```python
from build123d import *

# Parameters (mm, degrees)
SKETCH1_W           = 393.4
SKETCH1_H           = 150
BOSS_EXTRUDE1_DEPTH = 3.3
SKETCH2_R           = 2
CUT_EXTRUDE1_DEPTH  = 257.520622953
SKETCH3_R           = 2
CUT_EXTRUDE2_DEPTH  = 4
SKETCH4_R           = 2
CUT_EXTRUDE3_DEPTH  = 4
SKETCH6_W           = 29.5
SKETCH6_H           = 13
SKETCH6_W_2         = 121.579447476
SKETCH6_H_2         = 18.9
CUT_EXTRUDE4_DEPTH  = 10


with BuildPart() as part:
    # Sketch1 → Boss-Extrude1 (new body)
    with BuildSketch(Plane.XY):
        with Locations((27, -50.5)):
            Rectangle(SKETCH1_W, SKETCH1_H)
    extrude(amount=BOSS_EXTRUDE1_DEPTH)

    # Sketch2 → Cut-Extrude1 (cut, through all)
    with BuildSketch(Plane(origin=(0, 0, 0), x_dir=(-1, 0, 0), z_dir=(0, 0, -1))):
        with Locations((-183.7, -115.5)):
            Circle(SKETCH2_R)
        with Locations((-213.7, -115.5)):
            Circle(SKETCH2_R)
        with Locations((129.7, -115.5)):
            Circle(SKETCH2_R)
        with Locations((159.7, -115.5)):
            Circle(SKETCH2_R)
    extrude(amount=-CUT_EXTRUDE1_DEPTH, mode=Mode.SUBTRACT)

    # Sketch3 → Cut-Extrude2 (cut)
    with BuildSketch(Plane.XY.offset(3.3)):
        with Locations((-159.7, 14.5)):
            Circle(SKETCH3_R)
        with Locations((-139.7, 14.5)):
            Circle(SKETCH3_R)
        with Locations((193.7, 14.5)):
            Circle(SKETCH3_R)
        with Locations((213.7, 14.5)):
            Circle(SKETCH3_R)
    extrude(amount=-CUT_EXTRUDE2_DEPTH, mode=Mode.SUBTRACT)

    # Sketch4 → Cut-Extrude3 (cut)
    with BuildSketch(Plane.XY.offset(3.3)):
        with Locations((12, 12.25)):
            Circle(SKETCH4_R)
        with Locations((42, 12.25)):
            Circle(SKETCH4_R)
    extrude(amount=-CUT_EXTRUDE3_DEPTH, mode=Mode.SUBTRACT)

    # Sketch6 → Cut-Extrude4 (cut)
    with BuildSketch(Plane(origin=(0, 0, 0), x_dir=(-1, 0, 0), z_dir=(0, 0, -1))):
        with Locations((-36.8, -79)):
            Rectangle(SKETCH6_W, SKETCH6_H)
        with Locations((-27, -97.742382112)):
            Rectangle(SKETCH6_W_2, SKETCH6_H_2)
    extrude(amount=-CUT_EXTRUDE4_DEPTH, mode=Mode.SUBTRACT)


solid = part.part
```
Geometry: final body of the model. Coordinates: model frame, mm. Round coordinates to 2 decimals unless told otherwise and drop trailing zeros. Loops run counter-clockwise (first coordinate to the right, second up) from the corner with the lowest first, then second, coordinate; pieces in that order, holes last.
Item 1: Line query: L1, parallel to Y at x = 12, z = 1.7; L2, parallel to Y at x = -159.7, z = 2.4; L3, parallel to Y at x = 66, z = 0.9. Output: solid intervals per line, ascending.
Checked values:
L1: y = -125.5 to -107.19, -88.29 to 10.25, 14.25 to 24.5
L2: y = -125.5 to -117.5, -113.5 to 12.5, 16.5 to 24.5
L3: y = -125.5 to -107.19, -88.29 to 24.5
Item 2: Section B-B, the plane x = 80. Output: boundary loops of the cut face in (y, z), plus the area to 3 significant figures.
Checked values:
outline: (-125.5, 0) - (-107.19, 0) - (-107.19, 3.3) - (-125.5, 3.3) - close; (-88.29, 0) - (24.5, 0) - (24.5, 3.3) - (-88.29, 3.3) - close
area: 433 mm2
Item 3: Section A-A, the plane z = 2.75. State how many separate pieces and enclosed holes the cut face has, plus the area to 3 significant figures.
Checked values:
separate pieces: 1
enclosed holes: 12
area: 56,200 mm2
Item 4: Contact query for a flat-ended pin moving along its axis: P1, Ø3.5, axis at x = 42, y = 12.25, coming from the +Z side. Output: stop coordinate, or through.
Checked values:
P1: passes through
